Autodesk Inventor part; units mm, degrees
ref_plane "YZ Plane" through (0, 0, 0) normal (1, 0, 0) x (0, 1, 0)
ref_plane "XZ Plane" through (0, 0, 0) normal (0, 1, 0) x (-1, 0, 0)
ref_plane "XY Plane" through (0, 0, 0) normal (0, 0, 1) x (1, 0, 0)
sketch "Sketch1" plane through (0, 0, 0) normal (0, 0, 1) x (1, 0, 0)
  line L0 (-7.5576, 4.5871) -> (63.1052, 4.5871)
  line L1 (63.1052, 4.5871) -> (63.1052, -29.4489)
  line L2 (63.1052, -29.4489) -> (-7.5576, -29.4489)
  line L3 (-7.5576, -29.4489) -> (-7.5576, 4.5871)
  point P0 (0, 0)
  dimension "d0" = 70.6628
  dimension "d1" = 34.036
extrude "Extrusion1" add sketch "Sketch1" along normal blind 16.256
fillet "Fillet1" radius 3.175 12 edges at (27.7738, 4.5871, 16.256) (-7.5576, -12.4309, 16.256) (63.1052, -12.4309, 16.256) (27.7738, -29.4489, 16.256) (27.7738, 4.5871, 0) (27.7738, -29.4489, 0) (63.1052, -12.4309, 0) (-7.5576, -12.4309, 0) (-7.5576, -29.4489, 8.128) (-7.5576, 4.5871, 8.128) (63.1052, 4.5871, 8.128) (63.1052, -29.4489, 8.128)
properties part number "Battery"
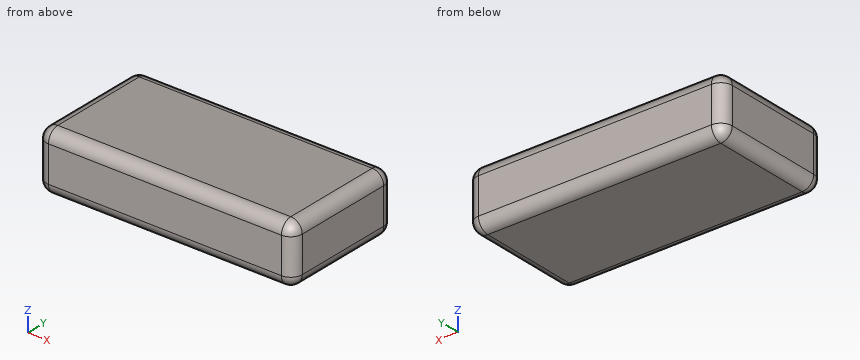
Can you work these out from the model? Positions are in its coordinate system, mm. Coordinates: 2 decimals unless noted, no trailing zeros. Loops run counter-clockwise (first coordinate to the right, second up) from the corner with the lowest first, then second, coordinate; pieces in that order, holes last. Notation, with made-up numbers: M 32.25,-7 L 87.25,-7 A33 ccw 87.25,22 Z; hole C 11.25,-35.5 d1. An arc over 180 degrees is marked long. Return JSON: item names as keys, results as strings. Group by question number.
Item 1: Imagine slicing it at A-A (x = 3.5). Please give me the cut outline in (y, z) (3 decimals), and give its area (3 significant figures).
Item 2: I'm going to push a flat-ended pin straight in: pin 1 Ø6 at (x, y) = (52.5, -14.5) entering from -Z. Where does the tip first touch, or does it pass through?
Item 3: If I drill on L1, parallel to X at y = -16, z = 13.25; L2, parallel to Y at x = 60, z = 6.25; L3, parallel to Y at x = 26.5, z = 14.25, over which ranges is the centre line in solid material (lowest first)? Write a range as from..to.
Verdict:
{
 "1": {"outline": "M -29.449,3.175 A3.175 ccw -26.274,0 L 1.412,0 A3.175 ccw 4.587,3.175 L 4.587,13.081 A3.175 ccw 1.412,16.256 L -26.274,16.256 A3.175 ccw -29.449,13.081 Z", "area": "545 mm^2"},
 "2": {"pin 1": "stops at z = 0"},
 "3": {"L1": "x = -7.55..63.1", "L2": "y = -29.45..4.59", "L3": "y = -29.23..4.36"}
}
